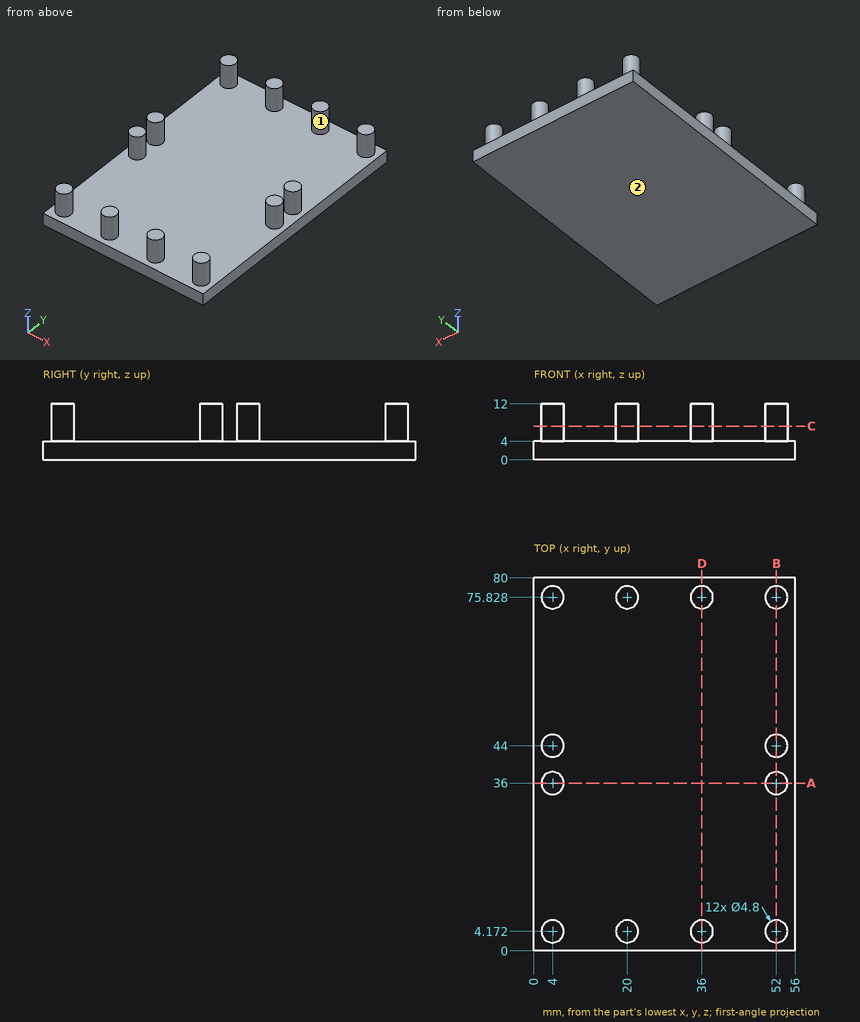
Source: three-view drawing plus pictorial views. Frame: mm from the lowest corner of the part. Give positions to 0.01 mm unless a question says otherwise; leave off trailing zeros. Order: outer loops, then holes, each group sorted by start corner. A loop starts at its lowest first (then second) coordinate and runs counter-clockwise, first axis right, second up.
1. Section B-B on x = 52. Return the cut outline in (y, z), and give its area (3 significant figures).
Derived:
outline: (0, 0) - (80, 0) - (80, 4) - (78.23, 4) - (78.23, 12) - (73.43, 12) - (73.43, 4) - (46.4, 4) - (46.4, 12) - (41.6, 12) - (41.6, 4) - (38.4, 4) - (38.4, 12) - (33.6, 12) - (33.6, 4) - (6.57, 4) - (6.57, 12) - (1.77, 12) - (1.77, 4) - (0, 4) - close
area: 474 mm2
2. Mould query, pull axis X, two halves, no side actions, for the marked faces 1 and 2. Classes: released by +X, released by -X, zero draft, split by the parting line, or undercut.
Derived:
face 1: undercut
face 2: zero draft
3. Material intervals for L1, parallel to X at y = 4.5, z = 8.5; L2, parallel to Z at x = 20, y = 62; L3, parallel to X at y = 77, z = 8.75 (1 decimal), sorted ascending.
Derived:
L1: x = 1.62 to 6.38, 17.62 to 22.38, 33.62 to 38.38, 49.62 to 54.38
L2: z = 0 to 4
L3: x = 1.9 to 6.1, 17.9 to 22.1, 33.9 to 38.1, 49.9 to 54.1
4. Pin query (flat end, axial travel): pin 1 (6 mm diameter, centred on x = 44, y = 18, fed in from +Z). Return the tip coordinate at first contact, or that it passes through.
Derived:
pin 1: stops at z = 4
5. Section D-D on x = 36. Return the cut outline in (y, z).
Derived:
outline: (0, 0) - (80, 0) - (80, 4) - (78.23, 4) - (78.23, 12) - (73.43, 12) - (73.43, 4) - (6.57, 4) - (6.57, 12) - (1.77, 12) - (1.77, 4) - (0, 4) - close
6. Section A-A on y = 36. Return the cut outline in (x, z).
Derived:
outline: (0, 0) - (56, 0) - (56, 4) - (54.4, 4) - (54.4, 12) - (49.6, 12) - (49.6, 4) - (6.4, 4) - (6.4, 12) - (1.6, 12) - (1.6, 4) - (0, 4) - close
7. Section C-C on z = 7.25. Give the number of separate pieces and of enclosed holes in the cut face, and give its area (3 significant figures).
Derived:
separate pieces: 12
enclosed holes: 0
area: 217 mm2
